```python
from build123d import *

# Parameters (mm, degrees)
SKETCH1_W           = 7.8
SKETCH1_H           = 60.325
BOSS_EXTRUDE1_DEPTH = 3
SKETCH2_W           = 2.5
SKETCH2_H           = 70.5
CUT_EXTRUDE1_DEPTH  = 3
SKETCH3_W           = 8
SKETCH3_H           = 3
BOSS_EXTRUDE2_DEPTH = 3


with BuildPart() as part:
    # Sketch1 → Boss-Extrude1 (new body)
    with BuildSketch(Plane.XY):
        Polygon((3, -10.75), (3, -0.75), (0, -0.75), (0, 19.25), (3, 19.25), (3, 29.25), (0, 29.25), (0, 42.5), (0, 44.5), (-21.311841589, 44.5), (-21.311841589, -26), (-19.311841589, -26), (-2, -26), (0, -26), (0, -24), (0, -10.75), align=None)
        with Locations((-7.4, 5.3775)):
            Rectangle(SKETCH1_W, SKETCH1_H, mode=Mode.SUBTRACT)
    extrude(amount=BOSS_EXTRUDE1_DEPTH)

    # Sketch2 → Cut-Extrude1 (cut)
    with BuildSketch(Plane.XY.offset(3)):
        with Locations((-20.061841589, 9.25)):
            Rectangle(SKETCH2_W, SKETCH2_H)
    extrude(amount=-CUT_EXTRUDE1_DEPTH, mode=Mode.SUBTRACT)

    # Sketch3 → Boss-Extrude2 (add)
    with BuildSketch(Plane.XY.offset(3)):
        with Locations((-10.655920795, -27.5)):
            Rectangle(SKETCH3_W, SKETCH3_H)
        with Locations((-10.655920795, 46)):
            Rectangle(SKETCH3_W, SKETCH3_H)
    extrude(amount=-BOSS_EXTRUDE2_DEPTH)


solid = part.part
```
Source: CAD feature listing. Evaluate the final solid. Frame: model axes, mm. A direction names the side the tool comes from. Coordinates: 2 decimals unless noted, no trailing zeros. Loops run counter-clockwise (first coordinate to the right, second up) from the corner with the lowest first, then second, coordinate; pieces in that order, holes last. Notation, with made-up numbers: M 35,6 L 49,6 A19 ccw 49,37 Z; hole C -12.5,5.25 d11. An arc over 180 degrees is marked long. Use a Markdown table: item, result. Add a question column.
Q1. Section query C-C, the plane z = 1.25. Return loops of the section in (x, y) (3 decimals), and give its area (3 significant figures).
Q2. Draft query along Y for faces 6 (the flat face through (-7, 35.54, 1)), 7 (the flat face through (0, 9, 1)), 8 (the flat face through (-17, -26, 1)), 9 (the flat face through (-6.656, 46, 2)). Return one class per face: pulls with the +Y half, pulls with the -Y half, needs draft (parallel to the pull), parting line crosses it, or undercut.
Q3. Material intervals for L1, parallel to Y at x = -6, z = 1.5 (3 decimals); L2, parallel to X at y = 15.5, z = 2; L3, parallel to X at y = 20.5, z = 0.9, sorted ascending.
Q4. Access query for faces 1 (the flat face through (-3, 44.5, 1)), 2 (the flat face through (-14.656, 46, 2)), 3 (the flat face through (-11.3, 5, 1)), 4 (the flat face through (1, 19.25, 1)), 5 (the flat face through (0, -18, 1)). Directions: +Z, -Z, +X, -X, +Y, -Y. A direction counts if a zero-diameter tool reaches every point of the face in a straight line with its end or side. Return the directions, or none.
Q5. First-contact query: pin 1 (0.9 mm diameter, centred on y = 45.5, z = 1.5, fed in from -X); pin 2 (1.5 mm diameter, centred on y = 9.5, z = 2, fed in from +X); pin 3 (1.5 mm diameter, centred on x = 1, z = 1, fed in from -Y). Flat tips, straight axial feed; report the tip coordinate or a pass-through.
Q6. Section query B-B, the plane x = -9. Return loops of the section in (y, z) (3 decimals).
Q7. Section query A-A, the plane y = -7.5. Return loops of the section in (x, z), and give its area (3 significant figures).
Result:
| question | item | result |
|---|---|---|
| 1 | outline | M -18.812,-26 L -14.656,-26 L -14.656,-29 L -6.656,-29 L -6.656,-26 L 0,-26 L 0,-10.75 L 3,-10.75 L 3,-0.75 L 0,-0.75 L 0,19.25 L 3,19.25 L 3,29.25 L 0,29.25 L 0,44.5 L -6.656,44.5 L -6.656,47.5 L -14.656,47.5 L -14.656,44.5 L -18.812,44.5 Z; hole M -11.3,-24.785 L -3.5,-24.785 L -3.5,35.54 L -11.3,35.54 Z |
| 1 | area | 964 mm2 |
| 2 | face 6 | undercut |
| 2 | face 7 | undercut |
| 2 | face 8 | pulls with the -Y half |
| 2 | face 9 | needs draft |
| 3 | L1 | y = -26 to -24.785, 35.54 to 44.5 |
| 3 | L2 | x = -18.81 to -11.3, -3.5 to 0 |
| 3 | L3 | x = -18.81 to -11.3, -3.5 to 3 |
| 4 | face 1 | +Z, -Z, +X, +Y |
| 4 | face 2 | +Z, -Z, -X, +Y |
| 4 | face 3 | +Z, -Z |
| 4 | face 4 | +Z, -Z, +X |
| 4 | face 5 | +Z, -Z, +X, -Y |
| 5 | pin 1 | stops at x = -14.66 |
| 5 | pin 2 | stops at x = 0 |
| 5 | pin 3 | stops at y = -10.75 |
| 6 | outline | M -29,0 L -24.785,0 L -24.785,3 L -29,3 Z; M 35.54,0 L 47.5,0 L 47.5,3 L 35.54,3 Z |
| 7 | outline | M -18.81,0 L -11.3,0 L -11.3,3 L -18.81,3 Z; M -3.5,0 L 3,0 L 3,3 L -3.5,3 Z |
| 7 | area | 42.0 mm2 |
